Build history of the part. All positions in model axes, mm. A direction names the side the tool comes from. Give positions to 0.01 mm unless a question says otherwise; leave off trailing zeros. Loops run counter-clockwise (first coordinate to the right, second up) from the corner with the lowest first, then second, coordinate; pieces in that order, holes last. Notation, with made-up numbers: M 56.25,19 L 64.25,19 A10 ccw 64.25,37 Z; hole C 19,53 d1. An arc over 180 degrees is marked long. Put each result on its own line as item: value.
```python
from build123d import *

# Parameters (mm, degrees)
SKETCH_1_R            = 35
EXTRUDE_1_DEPTH       = 90
SKETCH_3_R            = 30
CUT_EXTRUDE_1_DEPTH   = 80
EXTRUDE_START         = -4
EXTRUDE_3_OUTLINE_R   = 20
EXTRUDE_3_OUTLINE_R_2 = 12
EXTRUDE_3_DEPTH       = 8


# Read off the part's stored shape, not the designer's step: 凸台-拉伸3
with BuildPart() as part:
    # 草图1 → 凸台-拉伸1 (new body)
    with BuildSketch(Plane(origin=(0, 0, 0), x_dir=(1, 0, 0), z_dir=(0, 1, 0))):
        with Locations(Location((0, 0, 0), (0, 0, 90))):
            Circle(SKETCH_1_R)
    extrude(amount=EXTRUDE_1_DEPTH)

    # 草图3 → 切除-拉伸1 (cut)
    with BuildSketch(Plane(origin=(0, 90, 0), x_dir=(1, 0, 0), z_dir=(0, 1, 0))):
        with Locations(Location((0, 0, 0), (0, 0, 270))):
            Circle(SKETCH_3_R)
    extrude(amount=-CUT_EXTRUDE_1_DEPTH, mode=Mode.SUBTRACT)

    # 凸台-拉伸3 outline → 凸台-拉伸3 (add)
    with BuildSketch(Plane.XY.offset(EXTRUDE_START)):
        with Locations((50, 45)):
            Circle(EXTRUDE_3_OUTLINE_R)
        with Locations((50, 45)):
            Circle(EXTRUDE_3_OUTLINE_R_2, mode=Mode.SUBTRACT)
    extrude(amount=EXTRUDE_3_DEPTH)


solid = part.part
```
Q1. Tool access for faces 1 (the flat face through (60, 36, -4)), 2 (the flat face through (60, 36, 4)), 3 (the flat face through (0, 10, 0)): list every direction of +Z, -Z, +X, -X, +Y, -Y with a clear straight run to the whole face (end or side of a thin tool).
Here are the results:
face 1: -Z, +X, +Y, -Y
face 2: +Z, +X, +Y, -Y
face 3: +Y
Q2. Slice it at C-C (y = 69.5). List the corners of the cut face in (x, z), and give its area (3 significant figures).
Here are the results:
outline: C 0,0 d70; hole C 0,0 d60
area: 1,020 mm²
Q3. Mould opens along X. For faces 4 (the flat face through (0, 0, 0)), 5 (the cylindrical face through (69.99, 44.32, -0.06)) say: pulls with the +X half, pulls with the -X half, needs draft (parallel to the pull), parting line crosses it, or undercut.
Here are the results:
face 4: needs draft
face 5: undercut
Q4. Probe line 1 (Y direction, x = 50, z = -1.5); line 2 (X direction, y = 81, z = -0.5); line 3 (X direction, y = 40.5, z = 0). List the from-to ranges inside material, lowest first. Write a range as from..to.
Here are the results:
line 1: 25..33, 57..65
line 2: -35..-30, 30..35
line 3: -35..-30, 30..38.88, 61.12..69.49
Q5. Drop flat-ended pins along their axis: pin 1 Ø6 at (x, y) = (-16.5, 57.5) entering from +Z; pin 2 Ø1 at (y, z) = (62.5, -6.5) entering from -X; pin 3 Ø2 at (x, z) = (10.5, 26) entering from +Y. Give the stop position or say it passes through.
Here are the results:
pin 1: z = 32.29
pin 2: x = -34.48
pin 3: y = 10
Q6. Slice it at D-D (z = 0). List the corners of the cut face in (x, y).
Here are the results:
outline: M -35,0 L 35,0 L 35,31.77 A20 ccw long 35,58.23 L 35,90 L 30,90 L 30,10 L -30,10 L -30,90 L -35,90 Z; hole C 50,45 d24
Q7. Slice it at A-A (y = 45). List the corners of the cut face in (x, z).
Here are the results:
outline: M 34.77,-4 L 38,-4 L 38,4 L 34.77,4 A35 ccw long Z; M 62,-4 L 70,-4 L 70,4 L 62,4 Z; hole C 0,0 d60
Q8. Slice it at B-B (x = 50). List the corners of the cut face in (y, z).
Here are the results:
outline: M 25,-4 L 33,-4 L 33,4 L 25,4 Z; M 57,-4 L 65,-4 L 65,4 L 57,4 Z
